Autodesk Inventor part; units mm, degrees
ref_plane "YZ Plane" through (0, 0, 0) normal (1, 0, 0) x (0, 1, 0)
ref_plane "XZ Plane" through (0, 0, 0) normal (0, 1, 0) x (-1, 0, 0)
ref_plane "XY Plane" through (0, 0, 0) normal (0, 0, 1) x (1, 0, 0)
sketch "Sketch1" plane through (0, 0, 0) normal (0, 0, 1) x (1, 0, 0)
  line L0 (0, 0) -> (-156.6782, 0)
  line L1 (-156.6782, 0) -> (-156.6782, -1489.5)
  line L2 (-156.6782, -1489.5) -> (0, -1489.5)
  line L3 (0, -1489.5) -> (0, 0)
  line L4 (-156.6782, -1389.5) -> (-66, -1389.5)
  line L5 (-66, -1389.5) -> (-66, -1384.5)
  line L6 (-66, -1384.5) -> (-156.6782, -1384.5)
  line L7 (-156.6782, -1384.5) -> (-156.6782, -1389.5)
  line L8 (-156.6782, -892.8333) -> (-66, -892.8333)
  line L9 (-66, -892.8333) -> (-66, -887.8333)
  line L10 (-66, -887.8333) -> (-156.6782, -887.8333)
  line L11 (-156.6782, -887.8333) -> (-156.6782, -892.8333)
  line L12 (-156.6782, -396.1667) -> (-66, -396.1667)
  line L13 (-66, -396.1667) -> (-66, -391.1667)
  line L14 (-66, -391.1667) -> (-156.6782, -391.1667)
  line L15 (-156.6782, -391.1667) -> (-156.6782, -396.1667)
  circle A0 centre (-156.6782, -154.5) radius 30
  point P0 (-156.6782, -1384.5)
  point P1 (-156.6782, -124.5)
  point P2 (-156.6782, -184.5)
  dimension "d0" = 1489.5
  dimension "d1" = 156.6782
  dimension "d2" = 5
  dimension "d4" = 100
  dimension "d7" = 496.6667
  dimension "d23" = 66
  dimension "d28" = 60
  dimension "d29" = 1335
extrude "Plate1" add sketch "Sketch1" along normal blind 4 contours L3 L2 L1 L4 L5 L6 L8 L9 L10 L12 L13 L14 A0 L0
sketch "Sketch2" plane through (-4, 0, 0) normal (1, 0, 0) x (0, 1, 0)
  line L0 (-1489.5, 0) -> (0, 0)
  line L1 (0, 0) -> (0, 60)
  line L2 (0, 60) -> (-1489.5, 60)
  line L3 (-1489.5, 60) -> (-1489.5, 0)
edge flange "Flange1" height 60 angle 90 thickness 4 bend radius 4 thickness toward (1, 0, 0) relief tear relief width 4 relief depth 2 edges at (0, -744.75, 4) wall of the first edge with corners at (-4, -1489.5, 0) (-4, 0, 0) (-4, 0, 60) (-4, -1489.5, 60)
bend "Bend1"
corner "Corner1"
chamfer "Corner Chamfer1" distance 3 angle 45 6 edges at (-156.6782, -1389.5, 2) (-156.6782, -1384.5, 2) (-156.6782, -892.8333, 2) (-156.6782, -887.8333, 2) (-156.6782, -391.1667, 2) (-156.6782, -396.1667, 2)
sketch "Sketch4" plane through (0, -1489.5, 60) normal (1, 0, 0) x (0, 0, -1)
  circle A0 centre (18, 1059.5) radius 9
  line L0 (0, 0) -> (0, 1489.5)
  circle A1 centre (18, 562.8333) radius 9
  circle A2 centre (18, 66.1667) radius 9
  point P0 (60, 1489.5)
  dimension "d30" = 18
  dimension "d31" = 18
  dimension "d32" = 430
  dimension "d35" = 496.6667
extrude "Cut1" cut sketch "Sketch4" against normal blind 4
equation "\"d0\" = Стрингер_длина"
equation "\"d1\" = стрингер_глубина_4"
equation "\"d2\" = паз_под_стрингер_толщина"
equation "\"d7\" = Шаг_шпангоутов"
equation "\"d23\" = паз_под_стрингер_глубина - Thickness"
equation "\"d28\" = 2 * радиус_выреза_под_сварку"
equation "\"d35\" = Шаг_шпангоутов"
equation "\"d40\" = Thickness"
equation "\"d12\" = Thickness"
equation "\"d13\" = BendReliefWidth"
equation "\"d14\" = BendReliefDepth"
equation "\"d15\" = MinimumRemnant"
equation "\"d16\" = TransitionRadius"
equation "\"d17\" = ребро_усилителей"
equation "\"d19\" = BendRadius"
equation "\"d20\" = CornerReliefSize"
equation "\"d21\" = GapSize"
equation "\"d22\" = JacobiRadiusSize"
equation "\"BendRadius\" = Thickness"
equation "\"BendReliefWidth\" = Thickness"
equation "\"BendReliefDepth\" = 0.5 * Thickness"
equation "\"CornerReliefSize\" = 4 * Thickness"
equation "\"MinimumRemnant\" = 2 * Thickness"
equation "\"TransitionRadius\" = BendRadius"
equation "\"JacobiRadiusSize\" = BendRadius"
equation "\"GapSize\" = Thickness"
properties part number "GBK 0202 stringer 4" material "Steel"
Design review of the part built by this model. Coordinates are the model's own, in mm. A direction names the side the tool comes from. Round coordinates to 2 decimals unless told otherwise and drop trailing zeros. Write each loop counter-clockwise with the first axis right and the second up, starting at its lowest first coordinate (ties: lowest second). Pieces come first, ordered by that corner, then holes. Notation, with made-up numbers: (34, 45) - (60, 45) arc R20 cw to (60, 65) - close; hole circle Ø10 at (28, -37). An arc over 180 degrees is marked (long way). Use a Markdown table: item, result. Add a question column.
1. Clearance check with flat-ended pins moving along their axes: pin 1 (2 mm diameter, centred on y = -393.5, z = 3, fed in from -X); pin 2 (10 mm diameter, centred on y = -268, z = 33.5, fed in from -X); pin 3 (12 mm diameter, centred on x = -111.5, y = -584, fed in from +Z). State where each tip first meets the part, or that it passes through.
2. We need section A-A (x = -80). State the section outline as (y, z) points.
3. We need section C-C (y = -308). State the section outline as (x, z) points.
4. Wall thickness on probe 1 along Y at (x, z) = (-1.1, 42); probe 2 along X at (y, z) = (-811, 37.5); probe 3 along Z at (x, y) = (-50, -981): over which ranges is each line inside the solid? List them lowest first.
5. We need section D-D (y = -154.5). State the section outline as (x, z) points.
6. We need section B-B (z = 42). State the section outline as (x, y) points, then the cut area to 3 significant figures.
7. For faces 1 (the face through (-83, -734, 4)), 2 (the face through (-83, -734, 0)), list the 3-axis set-ups (+Z, -Z, +X, -X, +Y, -Y) from which the entire face can be reached by the end or side of a thin tool; tool diameter is ignored.
8. Mouldability with a two-part tool opening along Y and no side actions: class faces 3 (the face through (-55, -1489.5, 3)), 4 (the face through (-55, 0, 3)), 5 (the face through (-126.685, -153.84, 1.972)), 6 (the face through (-4, -734, 34)) as +Y half, -Y half, draft (parallel to the pull), parting line (faces both ways), or undercut.
Output:
| question | item | result |
|---|---|---|
| 1 | pin 1 | stops at x = -66 |
| 1 | pin 2 | stops at x = -4 |
| 1 | pin 3 | stops at z = 4 |
| 2 | outline | (-1489.5, 0) - (-1389.5, 0) - (-1389.5, 4) - (-1489.5, 4) - close; (-1384.5, 0) - (-892.83, 0) - (-892.83, 4) - (-1384.5, 4) - close; (-887.83, 0) - (-396.17, 0) - (-396.17, 4) - (-887.83, 4) - close; (-391.17, 0) - (0, 0) - (0, 4) - (-391.17, 4) - close |
| 3 | outline | (-156.68, 0) - (-8, 0) arc R8 ccw to (0, 8) - (0, 60) - (-4, 60) - (-4, 8) arc R4 cw to (-8, 4) - (-156.68, 4) - close |
| 4 | probe 1 | y = -1489.5 to -1432.33, -1414.33 to -935.67, -917.67 to -439, -421 to 0 |
| 4 | probe 2 | x = -4 to 0 |
| 4 | probe 3 | z = 0 to 4 |
| 5 | outline | (-126.68, 0) - (-8, 0) arc R8 ccw to (0, 8) - (0, 60) - (-4, 60) - (-4, 8) arc R4 cw to (-8, 4) - (-126.68, 4) - close |
| 6 | outline | (-4, -1489.5) - (0, -1489.5) - (0, -1432.33) - (-4, -1432.33) - close; (-4, -1414.33) - (0, -1414.33) - (0, -935.67) - (-4, -935.67) - close; (-4, -917.67) - (0, -917.67) - (0, -439) - (-4, -439) - close; (-4, -421) - (0, -421) - (0, 0) - (-4, 0) - close |
| 6 | area | 5,740 mm2 |
| 7 | face 1 | +Z, -X, +Y, -Y |
| 7 | face 2 | -Z, +X, -X, +Y, -Y |
| 8 | face 3 | -Y half |
| 8 | face 4 | +Y half |
| 8 | face 5 | undercut |
| 8 | face 6 | draft |
